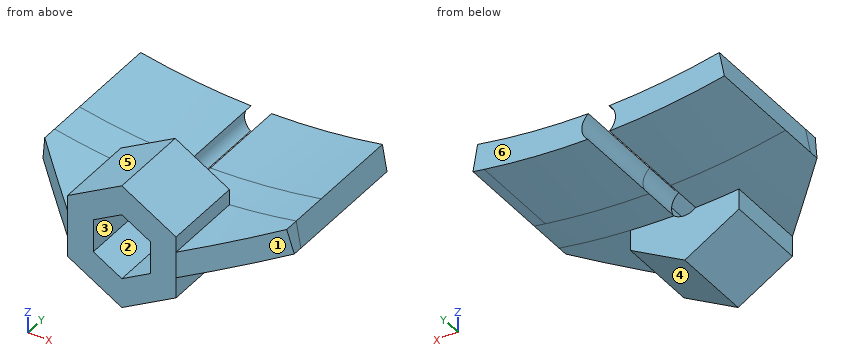
```python
from build123d import *

# Parameters (mm, degrees)
BOSS_EXTRUDE1_DEPTH     = 7
BOSS_EXTRUDE3_DEPTH     = 15
BOSS_EXTRUDE4_DEPTH     = 1
CUT_EXTRUDE1_DEPTH      = 33.699933964
CUT_EXTRUDE1_DEPTH_BACK = 33.699933964
SKETCH2_R               = 3.1
BOSS_EXTRUDE5_DEPTH     = 17.2
CUT_EXTRUDE3_DEPTH      = 37.841358298
CUT_EXTRUDE3_DEPTH_BACK = 37.841358298
CHAMFER1_SIZE           = 15


with BuildPart() as part:
    # Sketch1 → Boss-Extrude1 (new body)
    with BuildSketch(Plane(origin=(0, 0, 0), x_dir=(1, 0, 0), z_dir=(0, 1, 0))):
        with BuildLine():
            Line((-26.590677944, 0.897790933), (-24.677260394, -3.721607667))
            ThreePointArc((-24.677260394, -3.721607667), (-0.012479526, -1.099035349), (24.643498383, -3.80311637))
            Line((24.643498383, -3.80311637), (26.537632348, 0.769727537))
            ThreePointArc((26.537632348, 0.769727537), (26.536056466, 0.805424146), (26.507677261, 0.827134789))
            ThreePointArc((26.507677261, 0.827134789), (-0.03768972, 3.726158505), (-26.590677944, 0.897790933))
        make_face()
    extrude(amount=BOSS_EXTRUDE1_DEPTH)

    # Sketch1<4> → Boss-Extrude3 (add)
    with BuildSketch(Plane(origin=(0, 0, 0), x_dir=(1, 0, 0), z_dir=(0, 1, 0))):
        Polygon((0, 12.892692804), (-10, 7.119190112), (-10, -4.427815272), (0, -10.201317964), (10, -4.427815272), (10, 7.119190112), align=None)
        Polygon((0, 7.407865247), (-5.25, 4.376776333), (-5.25, -1.685401493), (0, -4.716490406), (5.25, -1.685401493), (5.25, 4.376776333), align=None, mode=Mode.SUBTRACT)
    extrude(amount=-BOSS_EXTRUDE3_DEPTH)

    # Sketch1<5> → Boss-Extrude4 (add)
    with BuildSketch(Plane(origin=(0, 0, 0), x_dir=(1, 0, 0), z_dir=(0, 1, 0))):
        Polygon((0, 12.892692804), (-10, 7.119190112), (-10, -4.427815272), (0, -10.201317964), (10, -4.427815272), (10, 7.119190112), align=None)
    extrude(amount=-BOSS_EXTRUDE4_DEPTH)

    # Sketch2 → Cut-Extrude1 (cut, two sides: drawn at the far end of the back side and taken through both)
    with BuildSketch(Plane.XZ.offset(1).offset(-CUT_EXTRUDE1_DEPTH_BACK)):
        with Locations(Location((0, -1.34568742, 0), (0, 0, 229.79522624))):
            Circle(SKETCH2_R)
    extrude(amount=CUT_EXTRUDE1_DEPTH + CUT_EXTRUDE1_DEPTH_BACK, mode=Mode.SUBTRACT)

    # Sketch3 → Boss-Extrude5 (add)
    with BuildSketch(Plane(origin=(0, 7, 0), x_dir=(1, 0, 0), z_dir=(0, 1, 0))):
        with BuildLine():
            ThreePointArc((-1.890425019, -1.111199481), (-12.112919314, -1.714534324), (-22.241796383, -3.220937936))
            Line((-22.241796383, -3.220937936), (-23.176627213, 1.588349763))
            ThreePointArc((-23.176627213, 1.588349763), (-12.634359148, 3.104112575), (-2.001116102, 3.713288389))
            ThreePointArc((-2.001116102, 3.713288389), (-3.099184389, 1.274580997), (-1.890425019, -1.111199481))
        make_face()
        with BuildLine():
            Line((22.31208714, -3.314700634), (23.163482432, 1.513802008))
            ThreePointArc((23.163482432, 1.513802008), (22.130674577, 1.706638646), (21.096276164, 1.890752624))
            ThreePointArc((21.096276164, 1.890752624), (11.587641271, 3.166667106), (2.008990202, 3.706610623))
            ThreePointArc((2.008990202, 3.706610623), (3.098925579, 1.264077023), (1.881941585, -1.117703712))
            ThreePointArc((1.881941585, -1.117703712), (12.145968264, -1.760973798), (22.31208714, -3.314700634))
        make_face()
    extrude(amount=BOSS_EXTRUDE5_DEPTH)

    # Sketch4 → Cut-Extrude3 (cut, two sides: drawn at the far end of the back side and taken through both)
    with BuildSketch(Plane(origin=(0, 7, 0), x_dir=(1, 0, 0), z_dir=(0, 1, 0)).offset(-CUT_EXTRUDE3_DEPTH_BACK)):
        with BuildLine():
            Line((23.163482432, 1.513802008), (22.31208714, -3.314700634))
            ThreePointArc((22.31208714, -3.314700634), (23.479051904, -3.552898091), (24.643498383, -3.80311637))
            Line((24.643498383, -3.80311637), (26.537632348, 0.769727537))
            ThreePointArc((26.537632348, 0.769727537), (26.536056466, 0.805424146), (26.507677261, 0.827134789))
            ThreePointArc((26.507677261, 0.827134789), (24.837933629, 1.181931749), (23.163482432, 1.513802008))
        make_face()
        with BuildLine():
            Line((-22.241796383, -3.220937936), (-23.176627213, 1.588349763))
            ThreePointArc((-23.176627213, 1.588349763), (-24.886067704, 1.255010478), (-26.590677944, 0.897790933))
            Line((-26.590677944, 0.897790933), (-24.677260394, -3.721607667))
            ThreePointArc((-24.677260394, -3.721607667), (-23.460875681, -3.464719015), (-22.241796383, -3.220937936))
        make_face()
    extrude(amount=CUT_EXTRUDE3_DEPTH + CUT_EXTRUDE3_DEPTH_BACK, mode=Mode.SUBTRACT)

    # Chamfer1
    # the kernel refuses this chamfer: 15 mm, written as the material it adds along each edge
    with BuildSketch(Plane(origin=(10, 0, 40.125691349), x_dir=(0.9996219169112966, 0.027495876610586365, 0), z_dir=(0, 0, -1))) as chamfer1_piece_1_section:
        Polygon((CHAMFER1_SIZE * 0.999621916911, CHAMFER1_SIZE * 0.0274958766106), (-CHAMFER1_SIZE * 0.0274958766106, CHAMFER1_SIZE * 0.999621916911), (0, 0), align=None)
    chamfer1_piece_1 = extrude(amount=82.008394033, mode=Mode.PRIVATE)
    chamfer1_piece_1 = chamfer1_piece_1 - Plane(origin=(-0.203357417, -3.100629743, 116.598877624), x_dir=(-0.21189526386996682, 0, -0.9772923805849901), z_dir=(0, -1, 0)) * Cylinder(115.5, 224, mode=Mode.PRIVATE)
    chamfer1_piece_1 = split(chamfer1_piece_1, bisect_by=Plane(origin=(22.567978143, -3.100629743, 1.863470638), z_dir=(-0.9848077530122092, 0, -0.17364817766692403)), keep=Keep.TOP, mode=Mode.PRIVATE)
    chamfer1_piece_1 = chamfer1_piece_1 & Plane(origin=(-0.203357417, -3.100629743, 120.773731271), x_dir=(0.21454646327949964, 0, -0.9767137836102542), z_dir=(0, -1, 0)) * Cylinder(124.5, 224, mode=Mode.PRIVATE)
    add(chamfer1_piece_1)
    with BuildSketch(Plane(origin=(-10, 0, -41.915476478), x_dir=(0.02749587661058632, -0.9996219169112968, 0), z_dir=(0, 0, 1))) as chamfer1_piece_2_section:
        Polygon((CHAMFER1_SIZE * 0.999621916911, -CHAMFER1_SIZE * 0.0274958766106), (-CHAMFER1_SIZE * 0.0274958766106, -CHAMFER1_SIZE * 0.999621916911), (0, 0), align=None)
    chamfer1_piece_2 = extrude(amount=82.005821637, mode=Mode.PRIVATE)
    chamfer1_piece_2 = chamfer1_piece_2 & Plane(origin=(-0.203357417, -2.670719626, 120.773731271), x_dir=(0.21454646327949964, 0, -0.9767137836102542), z_dir=(0, -1, 0)) * Cylinder(124.5, 224, mode=Mode.PRIVATE)
    chamfer1_piece_2 = chamfer1_piece_2 - Plane(origin=(-0.203357417, -2.670719626, 116.598877624), x_dir=(-0.21189526386996682, 0, -0.9772923805849901), z_dir=(0, -1, 0)) * Cylinder(115.5, 224, mode=Mode.PRIVATE)
    chamfer1_piece_2 = split(chamfer1_piece_2, bisect_by=Plane(origin=(-23.112985585, -2.670719626, -1.260941971), z_dir=(0.9816271834476646, 0, -0.1908089953765415)), keep=Keep.TOP, mode=Mode.PRIVATE)
    add(chamfer1_piece_2)


solid = part.part
```
Can you work these out from the model? Positions are in its coordinate system, mm. Face numbers are marked on the shaded views. A direction names the side the tool comes from. Round coordinates to 2 decimals unless told otherwise and drop trailing zeros. Loops run counter-clockwise (first coordinate to the right, second up) from the corner with the lowest first, then second, coordinate; pieces in that order, holes last. Notation, with made-up numbers: (29, 55) -> (71, 55) arc R12 ccw to (71, 73) -> close; hole circle Ø6 at (-33, 75). An arc over 180 degrees is marked (long way). One line per item, written item: value. Start each with the question number.
1. If we section it at D-D, the plane z = -8.25: Write out the boundary of the cut face in (x, y), then the cut area to 3 significant figures.
2. If we section it at B-B, the plane x = -1: Write out the boundary of the cut face in (y, z), then the cut area to 3 significant figures.
3. If I drill on probe 1 along X at (y, z) = (8, -0.5); probe 2 along Y at (x, z) = (-2.5, -6); probe 3 along Y at (x, z) = (-2, -5.25), over which ranges is the centre line in solid material (lowest first)?
4. For pin 1 (4 mm diameter, centred on y = 13.5, z = 2, fed in from -X); pin 2 (1.5 mm diameter, centred on y = -7.5, z = 3.5, fed in from -X); pin 3 (4 mm diameter, centred on x = -16, y = 10, fed in from -Z); pin 4 (3 mm diameter, centred on x = 0, z = -0.5, fed in from -Y), each with a flat end and sliding along its axis, tell me the tip position at first contact or that it passes through.
5. If we mould it in two halves opening along Z, with no side actions, what happens to the marked faces 3, 4, 5 and 6? For each: pulls with the +Z half, pulls with the -Z half, needs draft (parallel to the pull), parting line crosses it, or undercut.
6. For the marked faces 1 and 2, which set-ups out of +Z, -Z, +X, -X, +Y, -Y let a thin tool reach every point of the face, with its end or its side?
7. If we section it at C-C, the plane x = -15: Write out the boundary of the cut face in (y, z).
8. If we section it at A-A, the plane y = 21.5: Write out the boundary of the cut face in (x, z), then the cut area to 3 significant figures.
Calculated:
1. outline: (-8.04, -15) -> (8.04, -15) -> (8.04, 0) -> (-8.04, 0) -> close
1. area: 241 mm²
2. outline: (-15, -12.32) -> (0, -12.32) -> (0, -4.28) -> (-1, -4.28) -> (-1, -6.83) -> (-15, -6.83) -> close; (-15, 4.14) -> (-1, 4.14) -> (-1, 1.59) -> (0, 1.59) -> (0, 9.62) -> (-15, 9.62) -> close
2. area: 170 mm²
3. probe 1: x = -22.97 to -2.98, 2.98 to 22.98
3. probe 2: y = -15 to 0
3. probe 3: y = -1 to 0
4. pin 1: stops at x = -22.87
4. pin 2: stops at x = -10
4. pin 3: stops at z = -2.96
4. pin 4: passes through
5. face 3: undercut
5. face 4: pulls with the -Z half
5. face 5: pulls with the +Z half
5. face 6: needs draft
6. face 1: +Z, -Z, +X, -Y
6. face 2: -Y
7. outline: (-10, -2.84) -> (24.2, -2.84) -> (24.2, 2.05) -> (-10, 2.05) -> close
8. outline: (-23.18, -1.59) arc R124.5 ccw to (-2, -3.71) arc R3.1 cw to (-1.89, 1.11) arc R115.5 cw to (-22.24, 3.22) -> close; (1.88, 1.12) arc R3.1 cw to (2.01, -3.71) arc R124.5 ccw to (21.1, -1.89) arc R124.5 ccw to (23.16, -1.51) -> (22.31, 3.31) arc R115.5 cw to start
8. area: 195 mm²
